The listing builds one solid part. Answer for the finished solid, in the listing's coordinates (mm). Face numbers are marked on the shaded views. A direction names the side the tool comes from. Give positions to 0.01 mm unless a question says otherwise; leave off trailing zeros. Loops run counter-clockwise (first coordinate to the right, second up) from the corner with the lowest first, then second, coordinate; pieces in that order, holes last. Notation, with made-up numbers: M -35,5 L 13,5 A20 cw 13,18 Z; hole C 13.25,-31.5 d6. An arc over 180 degrees is marked long. Use one line per item in the form item = value. Start each with the question number.
1. The part is cut by section B-B (z = 8.75). Write down the section's boundary in (x, y) (3 decimals).
2. The part is cut by section D-D (y = 4.5). Write down the section's boundary in (x, z) (1 decimal), and give its area (3 significant figures).
3. Straight lines are drawn through the part: line 1 (X direction, y = -19, z = 6) (3 decimals); line 2 (Y direction, x = 5.5, z = 9.25); line 3 (X direction, y = -7, z = 3.5) (3 decimals). For each, find the intervals that lie inside material, in ascending order. Write a range as from..to.
4. The part is cut by section A-A (y = -19.5). Write down the section's boundary in (x, z) (3 decimals), and give its area (3 significant figures).
5. The part is cut by section C-C (x = 9.25). Write down the section's boundary in (y, z) (3 decimals).
6. Each of these flat-tipped pins is pushed along its axis until it touches: pin 1 Ø0.6 at (x, y) = (-10, -10) entering from -Z; pin 2 Ø3 at (y, z) = (12, 5.5) entering from +X; pin 3 Ø5 at (y, z) = (-7, 3) entering from +X (3 decimals). Where does it stop, or does it pass through?
7. The mould has two halves that part along X. Classify the marked faces 4, 5 and 6: released by +X, released by -X, zero draft, split by the parting line, or undercut.
8. For the marked faces 1, 2 and 3, determine the directions among +Z, -Z, +X, -X, +Y, -Y from which every point of the face is accessible in a straight line to the end or side of a thin tool.
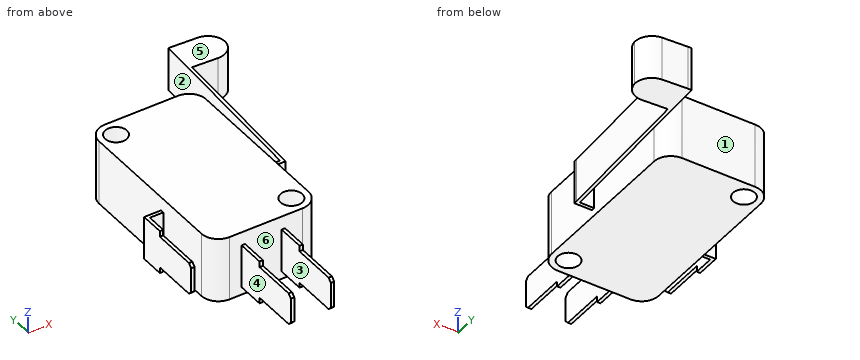
from build123d import *

# Parameters (mm, degrees)
F0_W         = 15.79
F0_H         = 27.86
F1_DEPTH     = 9.555
F2_R         = 2.5
F3_R         = 1.6
F4_DEPTH     = 25
F5_W         = 0.5
F5_H         = 6.4308560686
F6_DEPTH     = 4
F7_W         = 0.5
F7_H         = 4.7
F7_H_2       = 4.8242840722
F8_DEPTH     = 7
F9_SIZE      = 0.5
F10_W        = 0.5
F10_H        = 6.4308560686
F11_DEPTH    = 2.5
F12_W        = 0.5
F12_H        = 6.4308560686
F13_DEPTH    = 3
F14_W        = 0.5
F14_H        = 4.7
F15_DEPTH    = 7
F16_SIZE     = 0.5
F17_W        = 0.5
F17_H        = 6.4308560686
F18_DEPTH    = 2.6
F20_DEPTH    = 6.4308560686
F21_W        = 4.9
F21_H        = 6.4308560686
F22_DEPTH    = 6.2
F23_T1_DEPTH = 18.9308560686


# Not quite as in the source:
# - a fillet or chamfer that OpenCascade refuses, or shapes differently, is made with other operations: its cross-section is extruded or revolved along the edge and cut away or added


with BuildPart() as f1:
    # F0 (on Top) → F1 (new body)
    with BuildSketch(Plane.XY):
        Rectangle(F0_W, F0_H)
    extrude(amount=F1_DEPTH)

    # F2
    f2_edges = [f1.edges().sort_by_distance(p)[0] for p in [
        (-7.895, 13.93, 4.7775),
        (7.895, 13.93, 4.7775),
        (-7.895, -13.93, 4.7775),
        (7.895, -13.93, 4.7775),
    ]]
    fillet(f2_edges, radius=F2_R)

    # F3 (on face) → F4 (cut)
    with BuildSketch(Plane.XY.offset(9.555)):
        with Locations((-5.395, 11.43)):
            Circle(F3_R)
        with Locations((5.395, -11.43)):
            Circle(F3_R)
    extrude(amount=-F4_DEPTH, mode=Mode.SUBTRACT)

    # F5 (on face) → F6 (join)
    with BuildSketch(Plane.XZ.offset(13.93)):
        with Locations((-3.355, 4.3395719657)):
            Rectangle(F5_W, F5_H)
        with Locations((2.545, 4.3395719657)):
            Rectangle(F5_W, F5_H)
    extrude(amount=F6_DEPTH)

    # F7 (on face) → F8 (join)
    with BuildSketch(Plane.XZ.offset(17.93)):
        with Locations((-3.355, 4.3395719657)):
            Rectangle(F7_W, F7_H)
        with Locations((2.545, 4.2774299296)):
            Rectangle(F7_W, F7_H_2)
    extrude(amount=F8_DEPTH)

    # F9
    f9_edges = [f1.edges().sort_by_distance(p)[0] for p in [
        (-3.355, -24.93, 6.689572),
        (2.545, -24.93, 6.689572),
        (2.545, -24.93, 1.865288),
        (-3.355, -24.93, 1.989572),
    ]]
    chamfer(f9_edges, length=F9_SIZE)

    # F10 (on face) → F11 (join)
    with BuildSketch(Plane(origin=(-7.895, 0, 0), x_dir=(0, -1, 0), z_dir=(-1, 0, 0))):
        with Locations((2.68, 4.3395719657)):
            Rectangle(F10_W, F10_H)
    extrude(amount=F11_DEPTH)

    # F12 (on face) → F13 (join)
    with BuildSketch(Plane.XZ.offset(2.93)):
        with Locations((-10.145, 4.3395719657)):
            Rectangle(F12_W, F12_H)
    extrude(amount=F13_DEPTH)

    # F14 (on face) → F15 (join)
    with BuildSketch(Plane.XZ.offset(5.93)):
        with Locations((-10.145, 4.3395719657)):
            Rectangle(F14_W, F14_H)
    extrude(amount=F15_DEPTH)

    # F16
    f16_edges = [f1.edges().sort_by_distance(p)[0] for p in [
        (-10.145, -12.93, 6.689572),
        (-10.145, -12.93, 1.989572),
    ]]
    chamfer(f16_edges, length=F16_SIZE)

    # F17 (on face) → F18 (join)
    with BuildSketch(Plane.YZ.offset(7.895)):
        with Locations((-2.18, 4.3395719657)):
            Rectangle(F17_W, F17_H)
    extrude(amount=F18_DEPTH)

    # F19 (on face) → F20 (join, through all)
    with BuildSketch(Plane.XY.offset(7.555)):
        Polygon((11.3426885902, 25.0363132727), (9.9943753924, -1.93), (10.495, -1.93), (11.8433131978, 25.0363132727), align=None)
    extrude(amount=-F20_DEPTH)

    # F21 (on face) → F22 (join)
    with BuildSketch(Plane(origin=(10.5650872021, -0.528253394, 0), x_dir=(0.0499375258, 0.9987523434, 0), z_dir=(0.9987523434, -0.0499375258, 0))):
        with Locations((23.1465023109, 4.3395719657)):
            Rectangle(F21_W, F21_H)
    extrude(amount=F22_DEPTH)

    # F23: fillet of radius 2.5 on 2 edges, made by hand

    # F23_s2 → F23_t1 (cut)
    with BuildSketch(Plane.XY.offset(-5.1258560686)):
        with BuildLine():
            ThreePointArc((15.2940029919, 19.9576579442), (17.0961302855, 20.600699508), (17.9157276651, 22.3296949882))
            Line((17.9157276651, 22.3296949882), (17.7908838505, 19.8328141296))
            Line((17.7908838505, 19.8328141296), (15.2940029919, 19.9576579442))
        make_face()
        with BuildLine():
            ThreePointArc((15.5386968685, 24.8515444271), (17.2676923487, 24.0319470475), (17.9107339125, 22.2298197539))
            Line((17.9107339125, 22.2298197539), (18.0355777271, 24.7267006124))
            Line((18.0355777271, 24.7267006124), (15.5386968685, 24.8515444271))
        make_face()
    extrude(amount=F23_T1_DEPTH, mode=Mode.SUBTRACT)


solid = f1.part
Derived:
q1.outline = M -7.895,-11.43 A2.5 ccw -5.395,-13.93 L 5.395,-13.93 A2.5 ccw 7.895,-11.43 L 7.895,11.43 A2.5 ccw 5.395,13.93 L -5.395,13.93 A2.5 ccw -7.895,11.43 Z; hole C -5.395,11.43 d3.2; hole C 5.395,-11.43 d3.2
q2.outline = M -7.9,0 L 7.9,0 L 7.9,9.6 L -7.9,9.6 Z; M 10.3,1.1 L 10.8,1.1 L 10.8,7.6 L 10.3,7.6 Z
q2.area = 154 mm2
q3.line_1 = -3.605..-3.105, 2.295..2.795
q3.line_2 = -13.93..-13.03, -9.83..13.93
q3.line_3 = -10.395..-9.895, -7.895..7.895
q4.outline = M -3.605,1.99 L -3.105,1.99 L -3.105,6.69 L -3.605,6.69 Z; M 2.295,1.865 L 2.795,1.865 L 2.795,6.69 L 2.295,6.69 Z
q4.area = 4.76 mm2
q5.outline = M -2.43,1.124 L -1.93,1.124 L -1.93,7.555 L -2.43,7.555 Z
q6.pin_1 = 1.99
q6.pin_2 = 11.27
q6.pin_3 = 7.895
q7.face_4 = released by -X
q7.face_5 = zero draft
q7.face_6 = undercut
q8.face_1 = +Z, -Z, -X, +Y
q8.face_2 = +Z, -Z, +Y
q8.face_3 = +Z, -Z, -Y
